For this review, take the finished solid that the model builds, in its own axes (mm). A direction names the side the tool comes from. Coordinates: 2 decimals unless noted, no trailing zeros. Loops run counter-clockwise (first coordinate to the right, second up) from the corner with the lowest first, then second, coordinate; pieces in that order, holes last. Notation, with made-up numbers: (74.25, -26) - (80.25, -26) arc R23 cw to (80.25, -13) - close; hole circle Ø7 at (81.5, 88). An arc over 180 degrees is marked (long way). One line per item, written item: value. Start each with the question number.
1. Take a section at C-C, the plane y = -114.5. State the section outline as (x, z) points, and give its area (3 significant figures).
2. Take a section at A-A, the plane x = -16.5. State the section outline as (y, z) points.
3. Take a section at B-B, the plane z = 12.5. Count the separate pieces of the cut face and the enclosed holes in it, and give its area (3 significant figures).
4. For faces 4 (the face through (-50, -96.5, 13)), 5 (the face through (-5.7, -10, 12.3)), 6 (the face through (-7.05, -4.93, 15.2)), list the 3-axis set-ups (+Z, -Z, +X, -X, +Y, -Y) from which the entire face can be reached by the end or side of a thin tool; tool diameter is ignored.
5. Take a section at D-D, the plane y = -12.5. State the section outline as (x, z) points, and give its area (3 significant figures).
6. Insertion check: pin 1 (2 mm diameter, centred on x = -24.5, z = 4.5, fed in from -Y); pin 2 (1 mm diameter, centred on x = -40.5, z = 22.5, fed in from +Y); pin 3 (10 mm diameter, centred on y = -116, z = 3, fed in from +X). Each pin has a flat end and moves straight along its axis. Give the tip position at first contact, or say it passes through.
7. The part is to be moulded in two halves that separate along Y. For faces 1 (the face through (-29, -146.001, 12)), 2 (the face through (-5.7, -160, 12.3)), 3 (the face through (0, -5, 12)), say which applies: released by +Y, released by -Y, zero draft, split by the parting line, or undercut.
8. To check wall thickness, follow line 1 (Z direction, x = -10, y = -152); line 2 (Y direction, x = -18.5, z = 10.5); line 3 (Y direction, x = -46.5, z = 12.5). State the ranges of each line that lie inside material, in increasing order. Write a range as from..to.
```python
from build123d import *

# Parameters (mm, degrees)
BOSS_EXTRUDE1_DEPTH = 25
SKETCH3_R           = 10
CUT_EXTRUDE2_DEPTH  = 175.532828144
SKETCH4_R           = 4
CUT_EXTRUDE3_DEPTH  = 175.532828144


with BuildPart() as part:
    # Sketch1 → Boss-Extrude1 (new body)
    with BuildSketch(Plane.XY):
        Polygon((0, 0), (-20, 0), (-49.518324122, -30), (-65.09, -67.5), (-65.09, -92.5), (-49.518324122, -130), (-20, -160), (0, -160), (0, -150), (-20, -150), (-36.59, -130), (-36.59, -30), (-20, -10), (0, -10), align=None)
    extrude(amount=BOSS_EXTRUDE1_DEPTH)

    # Sketch3 → Cut-Extrude2 (cut, through all)
    with BuildSketch(Plane.ZY.offset(65.09)):
        with Locations((12.5, -80)):
            Circle(SKETCH3_R)
        with BuildLine():
            Line((6, -63.5), (19, -63.5))
            ThreePointArc((19, -63.5), (20.414213562, -62.914213562), (21, -61.5))
            Line((21, -61.5), (21, -15.999055713))
            ThreePointArc((21, -15.999055713), (20.414213562, -14.584842151), (19, -13.999055713))
            Line((19, -13.999055713), (6, -13.999055713))
            ThreePointArc((6, -13.999055713), (4.585786438, -14.584842151), (4, -15.999055713))
            Line((4, -15.999055713), (4, -61.5))
            ThreePointArc((4, -61.5), (4.585786438, -62.914213562), (6, -63.5))
        make_face()
        with BuildLine():
            Line((6, -146.000944287), (19, -146.000944287))
            ThreePointArc((19, -146.000944287), (20.414213562, -145.415157849), (21, -144.000944287))
            Line((21, -144.000944287), (21, -98.5))
            ThreePointArc((21, -98.5), (20.414213562, -97.085786438), (19, -96.5))
            Line((19, -96.5), (6, -96.5))
            ThreePointArc((6, -96.5), (4.585786438, -97.085786438), (4, -98.5))
            Line((4, -98.5), (4, -144.000944287))
            ThreePointArc((4, -144.000944287), (4.585786438, -145.415157849), (6, -146.000944287))
        make_face()
    extrude(amount=-CUT_EXTRUDE2_DEPTH, mode=Mode.SUBTRACT)

    # Sketch4 → Cut-Extrude3 (cut, through all)
    with BuildSketch(Plane(origin=(0, 0, 0), x_dir=(1, 0, 0), z_dir=(0, 1, 0))):
        with Locations(Location((-10, -12.5, 0), (0, 0, 180))):
            Circle(SKETCH4_R)
    extrude(amount=-CUT_EXTRUDE3_DEPTH, mode=Mode.SUBTRACT)


solid = part.part
```
Solutions:
1. outline: (-55.95, 0) - (-36.59, 0) - (-36.59, 4) - (-55.95, 4) - close; (-55.95, 21) - (-36.59, 21) - (-36.59, 25) - (-55.95, 25) - close
1. area: 155 mm2
2. outline: (-160, 0) - (-150, 0) - (-150, 25) - (-160, 25) - close; (-10, 0) - (0, 0) - (0, 25) - (-10, 25) - close
3. separate pieces: 6
3. enclosed holes: 0
3. area: 783 mm2
4. face 4: +X, -X, -Y
4. face 5: +Z, -Z, +X
4. face 6: +Y, -Y
5. outline: (-32.3, 0) - (-22.07, 0) - (-22.07, 25) - (-32.3, 25) - close
5. area: 256 mm2
6. pin 1: y = -156.44
6. pin 2: y = -20.33
6. pin 3: x = -36.59
7. face 1: undercut
7. face 2: released by -Y
7. face 3: zero draft
8. line 1: 0..8.5, 16.5..25
8. line 2: -160..-150, -10..0
8. line 3: -96.5..-90, -70..-63.5
